```python
from build123d import *

# Parameters (mm, degrees)
SKETCH1_R           = 72.5
SKETCH1_R_2         = 7
SKETCH1_R_3         = 2.5
SKETCH1_W           = 37
SKETCH1_H           = 36
SKETCH1_W_2         = 20
SKETCH1_H_2         = 20
BOSS_EXTRUDE1_DEPTH = 4


with BuildPart() as part:
    # Sketch1 → Boss-Extrude1 (new body)
    with BuildSketch(Plane(origin=(0, 0, 0), x_dir=(0, 0, -1), z_dir=(1, 0, 0))):
        Circle(SKETCH1_R)
        with Locations((-27.048330148, -18)):
            Circle(SKETCH1_R_2, mode=Mode.SUBTRACT)
        with Locations((0, 50)):
            Circle(SKETCH1_R_3, mode=Mode.SUBTRACT)
        with Locations((43.301270189, -25)):
            Circle(SKETCH1_R_3, mode=Mode.SUBTRACT)
        with Locations((-43.301270189, -25)):
            Circle(SKETCH1_R_3, mode=Mode.SUBTRACT)
        with Locations((5.251669852, 0)):
            Rectangle(SKETCH1_W, SKETCH1_H, mode=Mode.SUBTRACT)
        with Locations((-27.048330148, 0)):
            Rectangle(SKETCH1_W_2, SKETCH1_H_2, mode=Mode.SUBTRACT)
    extrude(amount=BOSS_EXTRUDE1_DEPTH)


solid = part.part
```
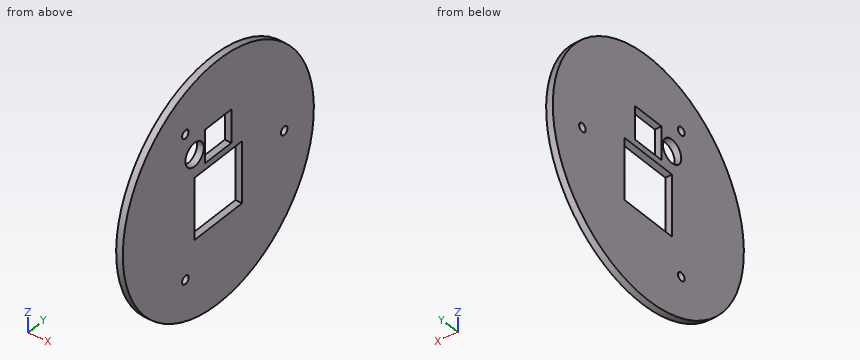
Geometry check sheet. Reference: the model listing, model coordinates, mm. Round coordinates to 2 decimals unless told otherwise and drop trailing zeros. Order: outer loops, then holes, each group sorted by start corner. A loop starts at its lowest first (then second) coordinate and runs counter-clockwise, first axis right, second up. Notation, with made-up numbers: (12, -27) -> (32, -27) arc R10 cw to (32, -12) -> close; hole circle Ø9 at (65, 35). An arc over 180 degrees is marked (long way). Return JSON: item names as keys, results as strings. Group by question number.
Q1. Gauge pin test, flat ends, axial feed: pin 1 (1.2 mm diameter, centred on x = 2.5, y = -2.5, fed in from -Z); pin 2 (2 mm diameter, centred on x = 1, y = -5, fed in from +Z); pin 3 (1 mm diameter, centred on x = 2.5, y = 47, fed in from +Z). Record the tip position at first contact, or that the pin passes through.
Q2. Section check B-B, the plane x = 1.45. Record the boundary of the cut face in (y, z), plus the area to 3 significant figures.
Q3. Section check C-C, the plane y = 50. Record the boundary of the cut face in (x, z).
Q4. Material ranges on probe 1 along Y at (x, z) = (2.8, 0); probe 2 along Z at (x, y) = (2.75, -13); probe 3 along Y at (x, z) = (1.85, -44.5), recorded low to high. Write a range as from..to.
Q5. Section check A-A, the plane z = 0. Record the boundary of the cut face in (x, y), plus the area to 3 significant figures.
Q6. Section check D-D, the plane y = 0. Record the boundary of the cut face in (x, z).
Numbers:
{
 "1": {"pin 1": "z = -72.48", "pin 2": "z = 72.39", "pin 3": "z = 55.62"},
 "2": {"outline": "circle Ø145 at (0, 0); hole circle Ø5 at (-25, -43.3); hole circle Ø5 at (-25, 43.3); hole circle Ø14 at (-18, 27.05); hole (-18, -23.75) -> (18, -23.75) -> (18, 13.25) -> (-18, 13.25) -> close; hole (-10, 17.05) -> (10, 17.05) -> (10, 37.05) -> (-10, 37.05) -> close; hole circle Ø5 at (50, 0)", "area": "14,600 mm^2"},
 "3": {"outline": "(0, -52.5) -> (4, -52.5) -> (4, -2.5) -> (0, -2.5) -> close; (0, 2.5) -> (4, 2.5) -> (4, 52.5) -> (0, 52.5) -> close"},
 "4": {"probe 1": "-72.5..-18, 18..47.5, 52.5..72.5", "probe 2": "-71.32..-23.75, 13.25..22.15, 31.95..71.32", "probe 3": "-57.24..-27.19, -22.81..57.24"},
 "5": {"outline": "(0, -72.5) -> (4, -72.5) -> (4, -18) -> (0, -18) -> close; (0, 18) -> (4, 18) -> (4, 47.5) -> (0, 47.5) -> close; (0, 52.5) -> (4, 52.5) -> (4, 72.5) -> (0, 72.5) -> close", "area": "416 mm^2"},
 "6": {"outline": "(0, -72.5) -> (4, -72.5) -> (4, -23.75) -> (0, -23.75) -> close; (0, 13.25) -> (4, 13.25) -> (4, 17.05) -> (0, 17.05) -> close; (0, 37.05) -> (4, 37.05) -> (4, 72.5) -> (0, 72.5) -> close"}
}
